The drawing under review shows one solid part. Ordinate dimensions are in mm from its lowest x, y, z. A direction names the side the tool comes from. Round coordinates to 2 decimals unless told otherwise and drop trailing zeros. Order: outer loops, then holes, each group sorted by start corner. A loop starts at its lowest first (then second) coordinate and runs counter-clockwise, first axis right, second up. Notation, with made-up numbers: M -4,20.5 L 20,20.5 A18 cw 20,39.5 Z; hole C 60,20 d5. An arc over 180 degrees is marked long. Answer as a JSON object with one key per item and string values.
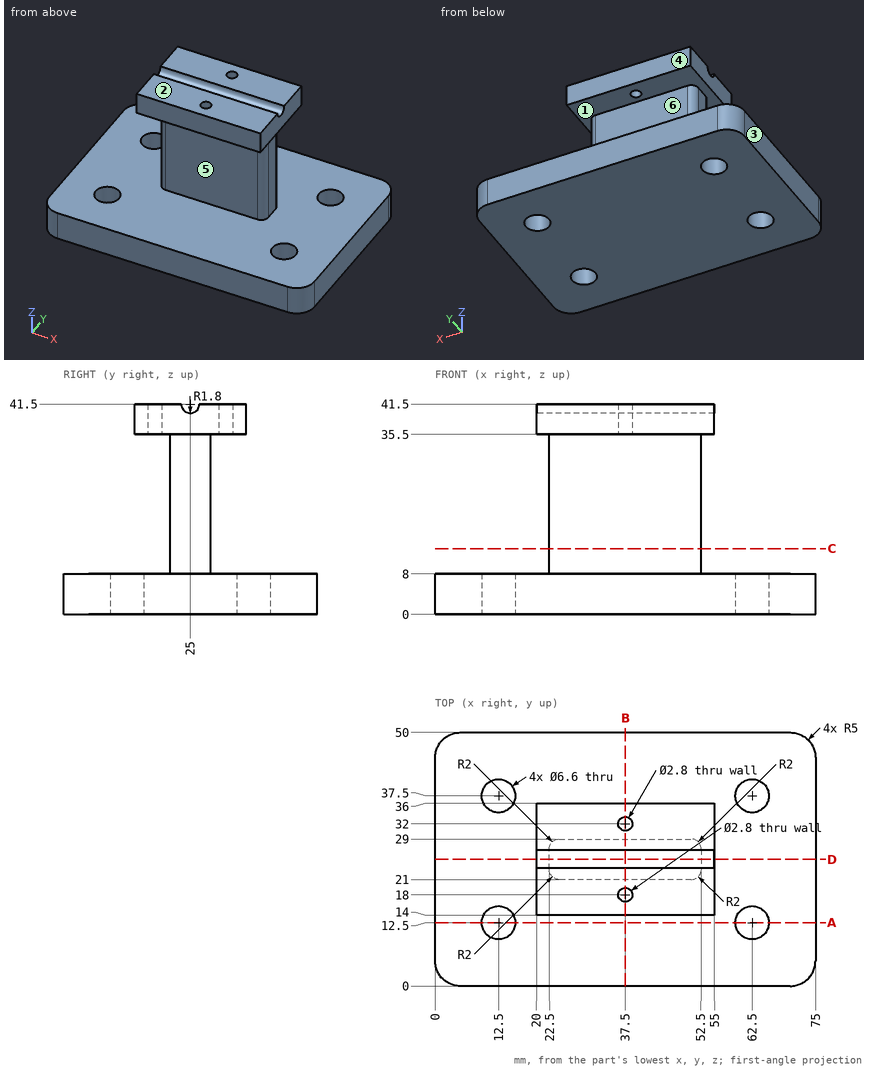
1) Add section D-D on y = 25. State the section outline as (x, z) points.
Geometry check:
{"outline": "M 0,0 L 75,0 L 75,8 L 52.5,8 L 52.5,35.5 L 55,35.5 L 55,39.7 L 20,39.7 L 20,35.5 L 22.5,35.5 L 22.5,8 L 0,8 Z"}
2) Insertion check: P1, Ø2, axis at x = 55, y = 12, coming from the +Z side; P2, Ø2, axis at y = 24, z = 29.5, coming from the -X side; P3, Ø21, axis at x = 34, z = 20.5, coming from the +Y side. Each pin has a flat end and moves straight along its axis. Give the tip position at first contact, or say it passes through.
Geometry check:
{"P1": "stops at z = 8", "P2": "stops at x = 22.5", "P3": "stops at y = 29"}
3) Add section B-B on x = 37.5. State the section outline as (y, z) points, and give its area (3 significant figures).
Geometry check:
{"outline": "M 0,0 L 50,0 L 50,8 L 29,8 L 29,35.5 L 30.6,35.5 L 30.6,41.5 L 26.8,41.5 A1.8 cw 23.2,41.5 L 19.4,41.5 L 19.4,35.5 L 21,35.5 L 21,8 L 0,8 Z; M 14,35.5 L 16.6,35.5 L 16.6,41.5 L 14,41.5 Z; M 33.4,35.5 L 36,35.5 L 36,41.5 L 33.4,41.5 Z", "area": "713 mm²"}
4) Machinability: for the marked faces 4, 5 and 6, which of the approach directions +Z, -Z, +X, -X, +Y, -Y give a long, thin tool a straight path to every point of the face, cutting with its end or side? Answer none if there is none.
Geometry check:
{"face 4": "+Z, +X, -X, +Y", "face 5": "+X, -X, -Y", "face 6": "+X, -X, +Y"}
5) Mouldability with a two-part tool opening along Z and no side actions: class the marked faces 1, 2 and 3 as +Z half, -Z half, draft (parallel to the pull), parting line (faces both ways), or undercut.
Geometry check:
{"face 1": "undercut", "face 2": "+Z half", "face 3": "draft"}
6) Add section A-A on y = 12.5. State the section outline as (x, z) points.
Geometry check:
{"outline": "M 0,0 L 9.2,0 L 9.2,8 L 0,8 Z; M 15.8,0 L 59.2,0 L 59.2,8 L 15.8,8 Z; M 65.8,0 L 75,0 L 75,8 L 65.8,8 Z"}
7) Add section C-C on z = 13. State the section outline as (x, y) points, and give its area (3 significant figures).
Geometry check:
{"outline": "M 22.5,23 A2 ccw 24.5,21 L 50.5,21 A2 ccw 52.5,23 L 52.5,27 A2 ccw 50.5,29 L 24.5,29 A2 ccw 22.5,27 Z", "area": "237 mm²"}
8) For L1, parallel to X at y = 12.5, z = 4; L2, parallel to X at y = 18, z = 39.9; L3, parallel to Y at x = 37, z = 38, list the stretches that pass through material, from the lowest coordinate up.
Geometry check:
{"L1": "x = 0 to 9.2, 15.8 to 59.2, 65.8 to 75", "L2": "x = 20 to 36.1, 38.9 to 55", "L3": "y = 14 to 16.69, 19.31 to 30.69, 33.31 to 36"}
